Can you work these out from the model? Positions are in its coordinate system, mm. Face numbers are marked on the shaded views. A direction names the side the tool comes from. Give positions to 0.01 mm unless a question says otherwise; leave off trailing zeros. Order: outer loops, then holes, each group sorted by start corner. A loop starts at its lowest first (then second) coordinate and runs counter-clockwise, first axis right, second up. Notation, with made-up numbers: M -9,33 L 12,33 A18 ccw 12,63 Z; hole C -21.75,60.5 d1. An arc over 180 degrees is marked long. Write each question's results on one line, items separated by ' | '.
from build123d import *

# Parameters (mm, degrees)
SALIENTE_EXTRUIR1_DEPTH    = 72.5
CORTAR_EXTRUIR1_DEPTH      = 31
CORTAR_EXTRUIR1_DEPTH_BACK = 140
CROQUIS2_W                 = 28
CROQUIS2_H                 = 55
CROQUIS2_W_2               = 22
CORTAR_EXTRUIR2_DEPTH      = 53
CORTAR_EXTRUIR2_DEPTH_BACK = 81
CROQUIS3_R                 = 2
CROQUIS5_R                 = 2
CORTAR_EXTRUIR3_DEPTH      = 81


with BuildPart() as part:
    # Croquis1 → Saliente-Extruir1 (new, symmetric)
    with BuildSketch(Plane.XY):
        with BuildLine():
            Line((-65.75, 14.5), (-64.25, 14.5))
            Line((-64.25, 14.5), (-64.25, -14))
            Line((-64.25, -14), (64.25, -14))
            Line((64.25, -14), (64.25, 14.5))
            Line((64.25, 14.5), (65.75, 14.5))
            Line((65.75, 14.5), (65.75, -14.5))
            ThreePointArc((65.75, -14.5), (65.457106781, -15.207106781), (64.75, -15.5))
            Line((64.75, -15.5), (-64.75, -15.5))
            ThreePointArc((-64.75, -15.5), (-65.457106781, -15.207106781), (-65.75, -14.5))
            Line((-65.75, -14.5), (-65.75, 14.5))
        make_face()
    extrude(amount=SALIENTE_EXTRUIR1_DEPTH, both=True)

    # Croquis2 → Cortar-Extruir1 (cut, two sides: drawn at the far end of the back side and taken through both)
    with BuildSketch(Plane.XZ.offset(15.5).offset(-CORTAR_EXTRUIR1_DEPTH_BACK)):
        with Locations((-51.75, -7)):
            Rectangle(CROQUIS2_W, CROQUIS2_H)
        with Locations((54.75, 15)):
            Rectangle(CROQUIS2_W_2, CROQUIS2_H)
    extrude(amount=CORTAR_EXTRUIR1_DEPTH + CORTAR_EXTRUIR1_DEPTH_BACK, mode=Mode.SUBTRACT)

    # Croquis3 → Cortar-Extruir2 (cut, two sides: drawn at the far end of the back side and taken through both)
    with BuildSketch(Plane.ZY.offset(65.75).offset(-CORTAR_EXTRUIR2_DEPTH_BACK)):
        with Locations(Location((59.5, -5.5, 0), (0, 0, 180))):
            Circle(CROQUIS3_R)
        with Locations(Location((-48.5, -6.5, 0), (0, 0, 180))):
            Circle(CROQUIS3_R)
    extrude(amount=CORTAR_EXTRUIR2_DEPTH + CORTAR_EXTRUIR2_DEPTH_BACK, mode=Mode.SUBTRACT)

    # Croquis5 → Cortar-Extruir3 (cut)
    with BuildSketch(Plane(origin=(65.75, 0, 0), x_dir=(0, 0, -1), z_dir=(1, 0, 0))):
        with Locations(Location((-54.5, -6.5, 0), (0, 0, 90))):
            Circle(CROQUIS5_R)
        with Locations(Location((57.5, -5.5, 0), (0, 0, 90))):
            Circle(CROQUIS5_R)
    extrude(amount=-CORTAR_EXTRUIR3_DEPTH, mode=Mode.SUBTRACT)


solid = part.part
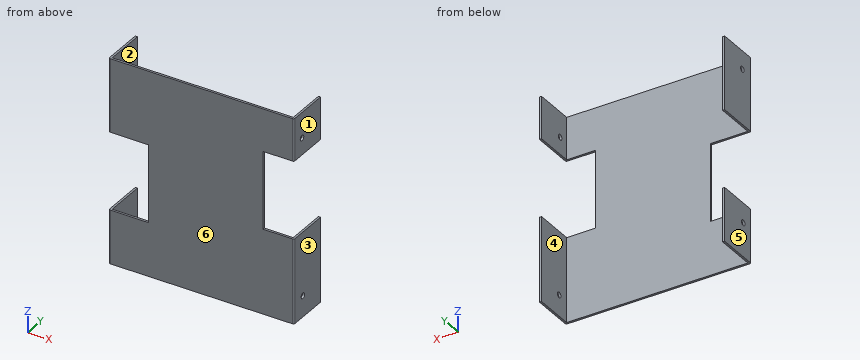
(1) I need wall thicknesses on L1, parallel to X at y = 5, z = -40; L2, parallel to Z at x = 65, y = -5; L3, parallel to Y at x = 48, z = -23. Which ranges of each line are inside material? Lowest first, please. Write a range as from..to.
Data:
L1: x = -65.75..-64.25, 64.25..65.75 | L2: z = -72.5..-59.44, -55.56..-12.5, 42.5..53.18, 55.82..72.5 | L3: y = -15.5..-14
(2) Imagine slicing it at C-C, the plane z = 40. Write out the boundary of the cut face in (x, y), plus the area to 3 significant figures.
Data:
outline: M -65.75,-14.5 A1 ccw -64.75,-15.5 L 43.75,-15.5 L 43.75,-14 L -64.25,-14 L -64.25,14.5 L -65.75,14.5 Z | area: 207 mm2
(3) Imagine slicing it at B-B, the plane y = 2. Write out the boundary of the cut face in (x, z).
Data:
outline: M -65.75,-72.5 L -64.25,-72.5 L -64.25,-34.5 L -65.75,-34.5 Z; M -65.75,20.5 L -64.25,20.5 L -64.25,72.5 L -65.75,72.5 Z; M 64.25,-72.5 L 65.75,-72.5 L 65.75,-12.5 L 64.25,-12.5 Z; M 64.25,42.5 L 65.75,42.5 L 65.75,72.5 L 64.25,72.5 Z
(4) Will these pins go through, and if not, where does the flat tip stop? P1, Ø3.5, axis at y = -6.5, z = -48.5, coming from the -X side; P2, Ø1.6, axis at y = -15, z = -16, coming from the -X side; P3, Ø10, axis at x = 45, z = -12, coming from the +Y side; P4, Ø12, axis at y = 1.5, z = 10, coming from the +X side.
Data:
P1: stops at x = 64.25 | P2: stops at x = -37.75 | P3: stops at y = -14 | P4: passes through
(5) For the marked faces 1 and 2, which set-ups out of +Z, -Z, +X, -X, +Y, -Y let a thin tool reach every point of the face, with its end or its side?
Data:
face 1: +Z, -Z, +X, +Y, -Y | face 2: +Z, -Z, +Y
(6) We'd pull the mould along X, two halves only. Please class the marked faces 3, 4, 5 and 6: +X half, -X half, draft (parallel to the pull), parting line (faces both ways), or undercut.
Data:
face 3: +X half | face 4: undercut | face 5: -X half | face 6: draft
(7) Imagine slicing it at D-D, the plane x = 20.5. Write out the boundary of the cut face in (y, z).
Data:
outline: M -15.5,-72.5 L -14,-72.5 L -14,72.5 L -15.5,72.5 Z
(8) Imagine slicing it at A-A, the plane z = -57.5. Write out the boundary of the cut face in (x, y).
Data:
outline: M -65.75,-14.5 A1 ccw -64.75,-15.5 L 64.75,-15.5 A1 ccw 65.75,-14.5 L 65.75,-7.5 L 64.25,-7.5 L 64.25,-14 L -64.25,-14 L -64.25,14.5 L -65.75,14.5 Z; M 64.25,-3.5 L 65.75,-3.5 L 65.75,14.5 L 64.25,14.5 Z
